from build123d import *

# Parameters (mm, degrees)
F0_W     = 882
F0_H     = 120
F1_DEPTH = 9
F3_DEPTH = 9.001


with BuildPart() as f1:
    # F0 (on Top) → F1 (new body)
    with BuildSketch(Plane.XY):
        with Locations((395.077364, 50.783694)):
            Rectangle(F0_W, F0_H)
    extrude(amount=F1_DEPTH)

    # F2 (on face) → F3 (cut, through all)
    with BuildSketch(Plane.XY.offset(9)):
        Polygon((770.077364, 104.783694), (767.077364, 104.783694), (767.077364, 99.783694), (755.077364, 99.783694), (755.077364, 77.783694), (767.077364, 77.783694), (767.077364, 35.783694), (836.077364, 35.783694), (836.077364, 110.783694), (770.077364, 110.783694), align=None)
        Polygon((-45.922636, 35.783694), (37.077364, 35.783694), (37.077364, 77.783694), (49.077364, 77.783694), (49.077364, 99.783694), (37.077364, 99.783694), (37.077364, 104.783694), (22.077364, 104.783694), (22.077364, 110.783694), (-45.922636, 110.783694), align=None)
    extrude(amount=-F3_DEPTH, mode=Mode.SUBTRACT)


solid = f1.part
For this review, take the finished solid that the model builds, in its own axes (mm). Coordinates: 2 decimals unless noted, no trailing zeros. Loops run counter-clockwise (first coordinate to the right, second up) from the corner with the lowest first, then second, coordinate; pieces in that order, holes last. Notation, with made-up numbers: (-9.75, 82.25) -> (33.25, 82.25) arc R23 ccw to (33.25, 112.25) -> close; hole circle Ø10 at (-35.5, 33.5). An arc over 180 degrees is marked (long way). Write each question's results on one line, items separated by ' | '.
Q1. Add section A-A, the plane z = 4.5. State the section outline as (x, y) points.
Taken from the geometry:
outline: (-45.92, -9.22) -> (836.08, -9.22) -> (836.08, 35.78) -> (767.08, 35.78) -> (767.08, 77.78) -> (755.08, 77.78) -> (755.08, 99.78) -> (767.08, 99.78) -> (767.08, 104.78) -> (770.08, 104.78) -> (770.08, 110.78) -> (22.08, 110.78) -> (22.08, 104.78) -> (37.08, 104.78) -> (37.08, 99.78) -> (49.08, 99.78) -> (49.08, 77.78) -> (37.08, 77.78) -> (37.08, 35.78) -> (-45.92, 35.78) -> close
Q2. Add section B-B, the plane y = 51.5. State the section outline as (x, z) points, then the cut area to 3 significant figures.
Taken from the geometry:
outline: (37.08, 0) -> (767.08, 0) -> (767.08, 9) -> (37.08, 9) -> close | area: 6,570 mm²
Q3. For pin 1 Ø2.5 at (y, z) = (59.5, 6.5) entering from +X; pin 2 Ø5 at (y, z) = (109, 2.5) entering from -X; pin 3 Ø3 at (y, z) = (65.5, 5.5) entering from -X, all flat-tipped, find the tip position at first contact; note any pin that passes through.
Taken from the geometry:
pin 1: x = 767.08 | pin 2: x = 22.08 | pin 3: x = 37.08
Q4. To check wall thickness, follow line 1 along X through (y, z) = (76, 6.25); line 2 along X through (y, z) = (79.5, 2.25). State the ranges of each line that lie inside material, in increasing order. Write a range as [from, to].
Taken from the geometry:
line 1: [37.08, 767.08] | line 2: [49.08, 755.08]
